Source: CAD feature listing. Evaluate the final solid. Frame: model axes, mm. Give positions to 0.01 mm unless a question says otherwise; leave off trailing zeros. Loops run counter-clockwise (first coordinate to the right, second up) from the corner with the lowest first, then second, coordinate; pieces in that order, holes last. Notation, with made-up numbers: M 21,3.5 L 50,3.5 A25 ccw 50,18.5 Z; hole C 63.25,13.25 d2. An arc over 180 degrees is marked long. Put each result on its own line as item: value.
from build123d import *

# Parameters (mm, degrees)
DIA_R = 0.8


with BuildPart() as part:
    # O-Ring: sweep along a path in FlowPath
    with BuildLine(Plane(origin=(0, 0, 0), x_dir=(1, 0, 0), z_dir=(0, 1, 0))) as o_ring_path:
        Line((-11.020937583, -1.724048364), (-1.305608269, -5.504904924))
        ThreePointArc((-1.305608269, -5.504904924), (0, -5.75), (1.305608269, -5.504904924))
        Line((1.305608269, -5.504904924), (11.020937583, -1.724048364))
        ThreePointArc((11.020937583, -1.724048364), (12.2, 0), (11.020937583, 1.724048364))
        Line((11.020937583, 1.724048364), (1.305608269, 5.504904924))
        ThreePointArc((1.305608269, 5.504904924), (0, 5.75), (-1.305608269, 5.504904924))
        Line((-1.305608269, 5.504904924), (-11.020937583, 1.724048364))
        ThreePointArc((-11.020937583, 1.724048364), (-12.2, 0), (-11.020937583, -1.724048364))
    # Dia → O-Ring (sweep)
    with BuildSketch(Plane(origin=(-1.305608269, 0, 5.504904924), x_dir=(0.3626689636627123, 0, -0.9319180343763149), z_dir=(0.9319180343763149, 0, 0.3626689636627123))):
        Circle(DIA_R)
    sweep(path=o_ring_path.line)


solid = part.part
1. Section query B-B (y = 0.25). Output: boundary loops of the cut face in (x, z).
Found:
outline: M -11.3,-2.43 L -1.58,-6.21 A4.36 ccw 1.58,-6.21 L 11.3,-2.43 A2.61 ccw 11.3,2.43 L 1.58,6.21 A4.36 ccw -1.58,6.21 L -11.3,2.43 A2.61 ccw Z; hole M -10.75,-1.02 L -1.03,-4.8 A2.84 ccw 1.03,-4.8 L 10.75,-1.02 A1.09 ccw 10.75,1.02 L 1.03,4.8 A2.84 ccw -1.03,4.8 L -10.75,1.02 A1.09 ccw Z
2. Material intervals for line 1 (Z direction, x = -1.5, y = -0.1); line 2 (Z direction, x = -11.25, y = 0.35); line 3 (X direction, y = -0.25, z = -0.25), sorted ascending. Write a range as from..to.
Found:
line 1: -6.28..-4.58, 4.58..6.28
line 2: -2.41..-0.68, 0.68..2.41
line 3: -12.95..-11.41, 11.41..12.95
3. Draft query along Z for faces 1 (the cylindrical face through (6.33, -0.49, -4.23)), 2 (the cylindrical face through (-6.385, 0.035, 4.386)). Return one class per face: pulls with the +Z half, pulls with the -Z half, needs draft (parallel to the pull), parting line crosses it, or undercut.
Found:
face 1: undercut
face 2: undercut
4. Section query A-A (z = 0). Output: boundary loops of the cut face in (x, y).
Found:
outline: C -12.2,0 d1.6; C 12.2,0 d1.6
